Design review of the part built by this model. Coordinates are the model's own, in mm. A direction names the side the tool comes from. Coordinates: 2 decimals unless noted, no trailing zeros. Order: outer loops, then holes, each group sorted by start corner. A loop starts at its lowest first (then second) coordinate and runs counter-clockwise, first axis right, second up. Notation, with made-up numbers: M -17.5,-13.75 L -7.5,-13.75 A31 cw -7.5,19.25 Z; hole C -11,-19 d9. An arc over 180 degrees is marked long. Answer in a Markdown table with one row per item.
from build123d import *

# Parameters (mm, degrees)
F3_SIZE = 3


# Not quite as in the source:
# - a fillet or chamfer that OpenCascade refuses, or shapes differently, is made with other operations: its cross-section is extruded or revolved along the edge and cut away or added


with BuildPart() as f1:
    # F0 (on Front) → F1 (revolve)
    with BuildSketch(Plane.XZ):
        Polygon((36.5, 7.6), (2, 7.6), (2, 8.25), (-3, 8.25), (-3, 0), (0, 0), (63.5, 0), (63.5, 4), (36.5, 4), align=None)
    revolve(axis=Axis((31.75, 0, 0), (-1, 0, 0)))

    # F2: fillet of radius 5 on 1 edges, made by hand

    # F2_s1 → F2_t2 (revolve)
    with BuildSketch(Plane.XZ):
        with BuildLine():
            ThreePointArc((41.3, 4), (38.3, 5), (36.5, 7.6))
            Line((36.5, 7.6), (36.5, 4))
            Line((36.5, 4), (41.3, 4))
        make_face()
    revolve(axis=Axis((36.5, 0, 0), (-1, 0, 0)))

    # F3
    f3_edges = [f1.edges().sort_by_distance(p)[0] for p in [
        (63.5, 0, -4),
    ]]
    chamfer(f3_edges, length=F3_SIZE)

    # F4: fillet of radius 8.1 on 1 edges, made by hand

    # F4_s1 → F4_t2 (revolve, cut)
    with BuildSketch(Plane.XZ):
        with BuildLine():
            ThreePointArc((2, 8.25), (-1.6349832962, 5.2666852265), (-3, 0.7666852265))
            Line((-3, 0.7666852265), (-3, 8.25))
            Line((-3, 8.25), (2, 8.25))
        make_face()
    revolve(axis=Axis((-3, 0, 0), (-1, 0, 0)), mode=Mode.SUBTRACT)


solid = f1.part
(1) Add section A-A, the plane x = 23. Give the boundary of the cut face in (y, z).
Return value:
| item | result |
|---|---|
| outline | C 0,0 d15.2 |
(2) Add section B-B, the plane x = 42.5. Give the boundary of the cut face in (y, z).
Return value:
| item | result |
|---|---|
| outline | C 0,0 d8 |
(3) Insertion check: pin 1 Ø1.5 at (y, z) = (-1, 3) entering from -X; pin 2 Ø4 at (x, y) = (54, -1.5) entering from +Z; pin 3 Ø4 at (y, z) = (-2.5, -5) entering from -X. Each pin has a flat end and moves straight along its axis. Give the tip position at first contact, or say it passes through.
Return value:
| item | result |
|---|---|
| pin 1 | stops at x = -2.83 |
| pin 2 | stops at z = 4 |
| pin 3 | stops at x = -2.49 |
(4) For faces 1 (the cylindrical face through (19.008, 0.334, -7.593)), 2 (the flat face through (-3, 0, 0)), list the 3-axis set-ups (+Z, -Z, +X, -X, +Y, -Y) from which the entire face can be reached by the end or side of a thin tool; tool diameter is ignored.
Return value:
| item | result |
|---|---|
| face 1 | +X |
| face 2 | +Z, -Z, -X, +Y, -Y |
(5) For line 1 along Z through (x, y) = (49, 1.25); line 2 along X through (y, z) = (-3.5, 4); line 3 along Z through (x, y) = (58, -0.5), list the stretches that pass through material, from the lowest coordinate up. Write a range as from..to.
Return value:
| item | result |
|---|---|
| line 1 | z = -3.8..3.8 |
| line 2 | x = -1.6..37.92 |
| line 3 | z = -3.97..3.97 |
